Autodesk Inventor part; units mm, degrees
ref_plane "Work Plane1" through (104.775, 0, 0) normal (0, 0, -1) x (1, 0, 0)
ref_plane "YZ Plane" through (0, 0, 0) normal (1, 0, 0) x (0, 1, 0)
ref_plane "XZ Plane" through (0, 0, 0) normal (0, 1, 0) x (-1, 0, 0)
sketch "Sketch1" plane through (0, 0, 0) normal (0, 0, 1) x (1, 0, 0)
  line L0 (35, 0) -> (35, 2)
  line L1 (35, 2) -> (15, 2)
  line L2 (15, 2) -> (14.5706, 2)
  line L3 (0, 3.765) -> (0, 1.4434)
  line L4 (0, 1.4434) -> (1.5, 1.4434)
  line L5 (1.5, 1.4434) -> (2.3333, 0)
  line L6 (2.3333, 0) -> (35, 0)
  line L7 (0, 3.765) -> (0.715, 3.765)
  line L8 (0.715, 3.765) -> (2.48, 2)
  line L9 (14.5706, 2) -> (2.48, 2)
  line L10 (15, 2) -> (2.48, 2) construction
  line L11 (2.48, 2) -> (2.48, 2)
  line L12 (-7, 0) -> (42, 0)
  line L13 (0, -0.753) -> (0, 4.518)
  dimension "d0" = 35
  dimension "d1" = 20
  dimension "d2" = 1.5
  dimension "d3" = 4
  dimension "d6" = 2.48
  dimension "d7" = 45
  dimension "d8" = 2.8868
  dimension "d9" = 60
  dimension "d10" = 7.53
  dimension "d11" = 4
  dimension "d12" = 0.4294
revolve "Body" add sketch "Sketch1" angle 360 about axis through (2.3333, 0, 0) along (1, 0, 0) contours L6 L5 L4 L3 L7 L8 L9 L2 L1 L0
sketch "Sketch2" plane through (0, 0, 0) normal (-1, 0, 0) x (0, 0, 1)
  circle A0 centre (0, 0) radius 1.4434
  line L0 (0, -5.271) -> (0, 5.271)
  line L1 (-5.271, 0) -> (5.271, 0)
  line L2 (1.4434, 0) -> (0.7217, -1.25)
  line L3 (0.7217, -1.25) -> (-0.7217, -1.25)
  line L4 (-0.7217, -1.25) -> (-1.4434, 0)
  line L5 (-1.4434, 0) -> (-0.7217, 1.25)
  line L6 (-0.7217, 1.25) -> (0.7217, 1.25)
  line L7 (0.7217, 1.25) -> (1.4434, 0)
  point P0 (0, 1.4434)
extrude "Slot" add sketch "Sketch2" against normal up to next contours L7 A0 | A0 L2 | L6 L0 A0 | A0 L0 L3 | L0 L6 A0 | A0 L3 L0 | L4 A0 | A0 L5
thread "Thread"
chamfer "Chamfer1" distance 0.4294 distance2 0.4294 1 edges at (35, -2, 0) measured on face at (35, -0.292, -0.9006)
ref_plane "Work Plane1" through (104.775, 0, 0) normal (0, 0, -1) x (1, 0, 0)
equation "\"d15\" = GEL"
equation "\"d17\" = -0.5 * SPD + 0.5 * GD"
equation "\"d18\" = GUL"
equation "\"d0\" = NLG"
equation "\"d1\" = GEL"
equation "\"d2\" = INTI"
equation "\"d3\" = GD"
equation "\"d6\" = KOH"
equation "\"d7\" = 0.5 * SEWI"
equation "\"d8\" = 1.1547 * SW"
equation "\"d10\" = KOD"
equation "\"d11\" = BDM"
equation "\"d12\" = GAL"
equation "\"NLG\" = 35"
equation "\"INTI\" = 1.5"
equation "\"GEL\" = 20"
equation "\"GAL\" = 0.61345 * PTC"
equation "\"KOH\" = 2.48"
equation "\"KOD\" = 7.53"
equation "\"GUL\" = 0.61345 * PTC"
equation "\"SPD\" = NND - 1.2269 * PTC"
equation "\"BDM\" = NND"
equation "\"GD\" = NND"
equation "\"SEWI\" = 90deg"
equation "\"SW\" = 2.5"
equation "\"TOA\" = 30deg"
equation "\"GD1\" = THREADDIA - 1.2269 * PTC"
equation "\"EPV\" = 4.48"
equation "\"THREADDIA\" = 4"
equation "\"PTC\" = 0.7"
equation "\"NND\" = 4"
equation "\"E0\" = 1.155 * SW"
properties part number "DIN 7991 - M4  x  35" material "Steel, Mild"
Here's how the part is built. I have some questions about the finished solid (model axes, mm). A direction names the side the tool comes from. Give positions to 0.01 mm unless a question says otherwise; leave off trailing zeros. Write each loop counter-clockwise with the first axis right and the second up, starting at its lowest first coordinate (ties: lowest second). Pieces come first, ordered by that corner, then holes. Notation, with made-up numbers: (60.25, -13) -> (87.25, -13) arc R13 cw to (87.25, 4) -> close; hole circle Ø11 at (61.25, 34). An arc over 180 degrees is marked (long way). Use one line per item in the form item = value. Start each with the question number.
1. Thinking about a two-plate mould opening in Y: for faces 4 (the face through (1, -1.25, 0)), 5 (the face through (0, 0, 2)), 6 (the face through (2.37, -0.46, 2.06)), which applies, +Y half, -Y half, draft (parallel to the pull), parting line (faces both ways), or undercut?
2. Imagine slicing it at A-A on x = 7. List the corners of the cut face in (y, z) for me.
3. Will these pins go through, and if not, where does the flat tip stop? pin 1 Ø2 at (x, y) = (11, -2) entering from +Z; pin 2 Ø2 at (x, z) = (10, -1.5) entering from -Y; pin 3 Ø4 at (x, y) = (20.5, -3) entering from -Z.
4. On a 3-axis mill with a long thin cutter (end or side, diameter ignored), from which of +Z, -Z, +X, -X, +Y, -Y can I reach the whole of each face in a straight line? I mean faces 1 (the face through (35, 0, 0)), 2 (the face through (0.795, -0.616, 1.088)), 3 (the face through (18, 0, 2)). Say none if no direction works.
5. If I drill on L1, parallel to Y at x = 21.5, z = 1.25; L2, parallel to X at y = -1.25, z = 3.5; L3, parallel to Y at x = 30, z = 1.5, over which ranges is the centre line in solid material (lowest first)?
Entries:
q1.face_4 = undercut
q1.face_5 = draft
q1.face_6 = parting line
q2.outline = circle Ø4 at (0, 0)
q3.pin_1 = 1.73
q3.pin_2 = -1.94
q3.pin_3 = -1.73
q4.face_1 = +Z, -Z, +X, +Y, -Y
q4.face_2 = -X
q4.face_3 = +X
q5.L1 = -1.56 to 1.56
q5.L2 = 0 to 0.76
q5.L3 = -1.32 to 1.32
